from build123d import *

# Parameters (mm, degrees)
F0_R     = 3.556
F1_DEPTH = 1.0414
F3_DEPTH = 1.4224


with BuildPart() as f1:
    # F0 (on Top) → F1 (new body)
    with BuildSketch(Plane.XY):
        Circle(F0_R)
    extrude(amount=-F1_DEPTH)

    # F2 (on face) → F3 (join)
    with BuildSketch(Plane(origin=(0, 0, -1.0414), x_dir=(1, 0, 0), z_dir=(0, 0, -1))):
        Polygon((0.011627, -4.106099), (3.561799, -2.04298), (3.550172, 2.063119), (-0.011627, 4.106099), (-3.561799, 2.04298), (-3.550172, -2.063119), align=None)
    extrude(amount=F3_DEPTH)

    # F4 (on Right) → F5 (revolve)
    with BuildSketch(Plane.YZ):
        with BuildLine():
            Line((0.006052, -2.459678), (0.006052, -4.96768))
            Line((0.006052, -4.96768), (1.953649, -4.96768))
            ThreePointArc((1.953649, -4.96768), (2.816414, -3.850818), (3.054052, -2.459678))
            Line((3.054052, -2.459678), (0.006052, -2.459678))
        make_face()
    revolve(axis=Axis((0, 0.006052, -3.713679), (0, 0, -1)))


solid = f1.part
Here's how the part is built. I have some questions about the finished solid (model axes, mm). A direction names the side the tool comes from. Give positions to 0.01 mm unless a question says otherwise; leave off trailing zeros. Answer as a JSON object with one key per item and string values. Group by question number.
1) Please list where these lines run through material, in increasing order: L1, parallel to Z at x = -2.75, y = -1.5; L2, parallel to X at y = 1, z = -1.6; L3, parallel to X at y = -0.5, z = -3.15. Write a range as [from, to].
2) On a 3-axis mill with a long thin cutter (end or side, diameter ignored), from which of +Z, -Z, +X, -X, +Y, -Y can I reach the whole of each face in a straight line? I mean faces 1 (the flat face through (-3.2, 1.9, -1.041)), 2 (the flat face through (0, 3.8, -1.041)), 3 (the cylindrical face through (-0.77, -3.47, -0.51)), 4 (the flat face through (-3.2, -1.9, -1.041)). Say none if no direction works.
3) I'm going to push flat-ended pins straight in: pin 1 Ø1.5 at (x, y) = (2.5, 2.5) entering from -Z; pin 2 Ø1.4 at (x, y) = (2.5, -2) entering from +Z; pin 3 Ø1 at (x, z) = (-1.5, -4) entering from -Y; pin 4 Ø0.5 at (x, y) = (-3, -2.5) entering from +Z. Where does each tip first touch, or does it pass through?
Results found:
{
 "1": {"L1": "[-2.46, 0]", "L2": "[-3.55, 3.56]", "L3": "[-2.98, 2.98]"},
 "2": {"face 1": "+Z, -X, +Y", "face 2": "+Z, +Y", "face 3": "+Z", "face 4": "+Z, -X, -Y"},
 "3": {"pin 1": "z = -3.92", "pin 2": "z = 0", "pin 3": "y = -2.65", "pin 4": "z = -1.04"}
}
